Model file for the job. Use its own axes, mm. Face numbers are marked on the shaded views. A direction names the side the tool comes from. Round coordinates to 2 decimals unless told otherwise and drop trailing zeros. Loops run counter-clockwise (first coordinate to the right, second up) from the corner with the lowest first, then second, coordinate; pieces in that order, holes last. Notation, with made-up numbers: (63.25, -19.5) -> (109.25, -19.5) arc R30 cw to (109.25, 9.5) -> close; hole circle Ø10 at (19.5, 87). An arc over 180 degrees is marked (long way). Use a Markdown table: item, result.
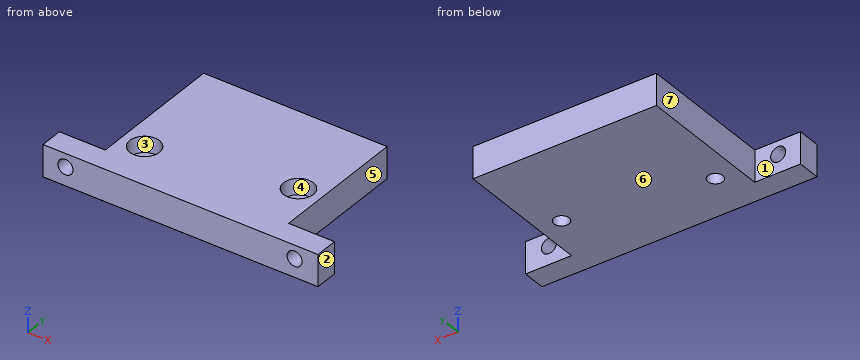
from build123d import *

# Parameters (mm, degrees)
SKETCH_1_W          = 60
SKETCH_1_H          = 6.9
EXTRUDE_1_DEPTH     = 5
SKETCH_2_R          = 1.65
CUT_EXTRUDE_1_DEPTH = 10
SKETCH_3_W          = 40
SKETCH_3_H          = 6.9
EXTRUDE_2_DEPTH     = 30
SKETCH_5_R          = 1.65
CUT_EXTRUDE_2_DEPTH = 25
CUT_EXTRUDE_START   = -3.5
SKETCH_6_R          = 3.25
SKETCH_6_R_2        = 1.65
CUT_EXTRUDE_3_DEPTH = 3.5


with BuildPart() as part:
    # 草图1 → 凸台-拉伸1 (new body)
    with BuildSketch(Plane(origin=(0, 0, 0), x_dir=(1, 0, 0), z_dir=(0, 1, 0))):
        with Locations((-12.970884588, 1.077948994)):
            Rectangle(SKETCH_1_W, SKETCH_1_H)
    extrude(amount=EXTRUDE_1_DEPTH)

    # 草图2 → 切除-拉伸1 (cut)
    with BuildSketch(Plane.XZ):
        with Locations(Location((11.923103363, -0.527948994, 0), (0, 0, 270))):
            Circle(SKETCH_2_R)
        with Locations(Location((-38.076896637, -0.527948994, 0), (0, 0, 270))):
            Circle(SKETCH_2_R)
    extrude(amount=-CUT_EXTRUDE_1_DEPTH, mode=Mode.SUBTRACT)

    # 草图3 → 凸台-拉伸2 (add)
    with BuildSketch(Plane(origin=(0, 5, 0), x_dir=(1, 0, 0), z_dir=(0, 1, 0))):
        with Locations((-12.970884588, 1.077948994)):
            Rectangle(SKETCH_3_W, SKETCH_3_H)
    extrude(amount=EXTRUDE_2_DEPTH)

    # 草图5 → 切除-拉伸2 (cut)
    with BuildSketch(Plane(origin=(0, 0, -4.527948994), x_dir=(-1, 0, 0), z_dir=(0, 0, -1))):
        with Locations((27.970884588, 10)):
            Circle(SKETCH_5_R)
        with Locations((-2.029115412, 15)):
            Circle(SKETCH_5_R)
    extrude(amount=-CUT_EXTRUDE_2_DEPTH, mode=Mode.SUBTRACT)

    # 草图6 → 切除-拉伸3 (cut)
    # profile 1 of 2: a face of its own
    with BuildSketch(Plane.XY.offset(2.372051006).offset(CUT_EXTRUDE_START)):
        with Locations((-27.970884588, 10)):
            Circle(SKETCH_6_R)
        with Locations(Location((-27.970884588, 10, 0), (0, 0, 180))):
            Circle(SKETCH_6_R_2, mode=Mode.SUBTRACT)
    # profile 2 of 2: a face of its own
    with BuildSketch(Plane.XY.offset(2.372051006).offset(CUT_EXTRUDE_START)):
        with Locations((2.029115412, 15)):
            Circle(SKETCH_6_R)
        with Locations(Location((2.029115412, 15, 0), (0, 0, 180))):
            Circle(SKETCH_6_R_2, mode=Mode.SUBTRACT)
    extrude(amount=CUT_EXTRUDE_3_DEPTH, mode=Mode.SUBTRACT)


solid = part.part
Q1. Band-saw the part on B-B, the plane y = 15. Give the cut face in (x, z).
Results list:
| item | result |
|---|---|
| outline | (-32.97, -4.53) -> (0.38, -4.53) -> (0.38, -1.13) -> (-1.22, -1.13) -> (-1.22, 2.37) -> (-32.97, 2.37) -> close; (3.68, -4.53) -> (7.03, -4.53) -> (7.03, 2.37) -> (5.28, 2.37) -> (5.28, -1.13) -> (3.68, -1.13) -> close |
Q2. Flat gauge pins, fed straight in: pin 1 (2 mm diameter, centred on y = 18.5, z = -3, fed in from +X); pin 2 (2 mm diameter, centred on y = 27, z = -1.5, fed in from -X). Where does each tip first touch, or does it go through?
Results list:
| item | result |
|---|---|
| pin 1 | stops at x = 7.03 |
| pin 2 | stops at x = -32.97 |
Q3. Band-saw the part on A-A, the plane z = 0.5. Give the cut face in (x, y), plus the area to 3 significant figures.
Results list:
| item | result |
|---|---|
| outline | (-42.97, 0) -> (-39.37, 0) -> (-39.37, 5) -> (-42.97, 5) -> close; (-36.79, 0) -> (10.63, 0) -> (10.63, 5) -> (7.03, 5) -> (7.03, 35) -> (-32.97, 35) -> (-32.97, 5) -> (-36.79, 5) -> close; (13.21, 0) -> (17.03, 0) -> (17.03, 5) -> (13.21, 5) -> close; hole circle Ø6.5 at (-27.97, 10); hole circle Ø6.5 at (2.03, 15) |
| area | 1,410 mm² |
Q4. Pull direction X, two halves, no side cores. Call the marked faces 1, 2, 3 and 4: released by +X, released by -X, zero draft, split by the parting line, or undercut.
Results list:
| item | result |
|---|---|
| face 1 | zero draft |
| face 2 | released by +X |
| face 3 | undercut |
| face 4 | undercut |
Q5. Band-saw the part on C-C, the plane x = 2. Give the cut face in (y, z), plus the area to 3 significant figures.
Results list:
| item | result |
|---|---|
| outline | (0, -4.53) -> (13.35, -4.53) -> (13.35, -1.13) -> (11.75, -1.13) -> (11.75, 2.37) -> (0, 2.37) -> close; (16.65, -4.53) -> (35, -4.53) -> (35, 2.37) -> (18.25, 2.37) -> (18.25, -1.13) -> (16.65, -1.13) -> close |
| area | 208 mm² |
Q6. Drill centre lines: L1, parallel to X at y = 10, z = -3.25; L2, parallel to X at y = 2, z = -1.25; L3, parallel to Y at x = -34, z = -1.25. Where is each one in solid material? Low to high. Write a range as from..to.
Results list:
| item | result |
|---|---|
| L1 | x = -32.97..-29.62, -26.32..7.03 |
| L2 | x = -42.97..-39.56, -36.59..10.44, 13.41..17.03 |
| L3 | y = 0..5 |
Q7. Band-saw the part on D-D, the plane z = -3.5. Give the cut face in (x, y).
Results list:
| item | result |
|---|---|
| outline | (-42.97, 0) -> (17.03, 0) -> (17.03, 5) -> (7.03, 5) -> (7.03, 35) -> (-32.97, 35) -> (-32.97, 5) -> (-42.97, 5) -> close; hole circle Ø3.3 at (-27.97, 10); hole circle Ø3.3 at (2.03, 15) |
Q8. Tool access for the marked faces 5, 6 and 7: list every direction of +Z, -Z, +X, -X, +Y, -Y with a clear straight run to the whole face (end or side of a thin tool).
Results list:
| item | result |
|---|---|
| face 5 | +Z, -Z, +X, +Y |
| face 6 | -Z, +X, -X, +Y, -Y |
| face 7 | +Z, -Z, -X, +Y |
